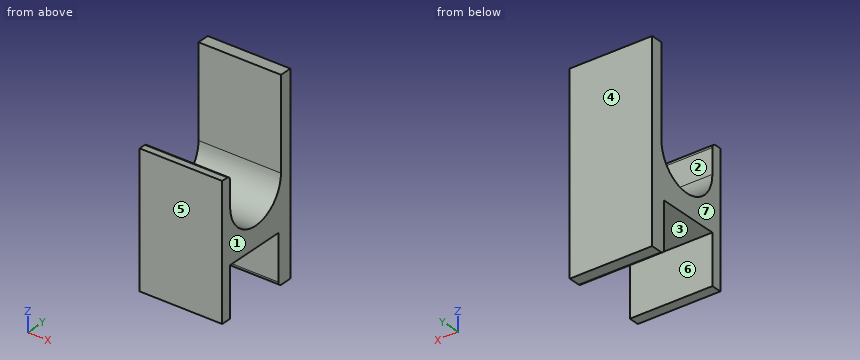
from build123d import *

# Parameters (mm, degrees)
F1_DEPTH = 25.4
F2_R     = 1.27
F3_R     = 1.27


with BuildPart() as f1:
    # F0 (on Right) → F1 (new body)
    with BuildSketch(Plane.YZ):
        with BuildLine():
            Line((-24.031516, -15.24), (-24.031516, 0))
            Line((-24.031516, 0), (-4.727516, 0))
            Line((-4.727516, 0), (-4.727516, -15.24))
            Line((-4.727516, -15.24), (0.022284, -15.24))
            Line((0.022284, -15.24), (0.022284, 44.45))
            Line((0.022284, 44.45), (-3.711516, 44.45))
            Line((-3.711516, 44.45), (-3.711516, 16.51))
            ThreePointArc((-3.711516, 16.51), (-13.871516, 6.35), (-24.031516, 16.51))
            Line((-24.031516, 16.51), (-24.031516, 25.4))
            Line((-24.031516, 25.4), (-27.206516, 25.4))
            Line((-27.206516, 25.4), (-27.206516, -15.24))
            Line((-27.206516, -15.24), (-26.082276, -15.24))
            Line((-26.082276, -15.24), (-24.031516, -15.24))
        make_face()
    extrude(amount=F1_DEPTH)

    # F2
    f2_edges = [f1.edges().sort_by_distance(p)[0] for p in [
        (12.7, -24.031516, 25.4),
    ]]
    fillet(f2_edges, radius=F2_R)

    # F3
    f3_edges = [f1.edges().sort_by_distance(p)[0] for p in [
        (12.7, -4.727516, -15.24),
    ]]
    fillet(f3_edges, radius=F3_R)


solid = f1.part
Model file for the job. Use its own axes, mm. Face numbers are marked on the shaded views. A direction names the side the tool comes from. Give positions to 0.01 mm unless a question says otherwise; leave off trailing zeros. Loops run counter-clockwise (first coordinate to the right, second up) from the corner with the lowest first, then second, coordinate; pieces in that order, holes last.
1) Saw through at D-D (z = 32.5). Write the cut outline in (x, y), plus the area to 3 significant figures.
2) Tool access for the marked faces 1, 2 and 3: list every direction of +Z, -Z, +X, -X, +Y, -Y with a clear straight run to the whole face (end or side of a thin tool).
3) Saw through at B-B (x = 16.5). Write the cut outline in (y, z).
4) Wall check: line 1 (Y direction, x = 2.75, z = -7.5); line 2 (Y direction, x = 24.5, z = 21); line 3 (Y direction, x = 8.25, z = 40.5). Give the ranges that are in metal, low to high.
5) Saw through at A-A (z = 20.5). Write the cut outline in (x, y).
6) Saw through at C-C (y = -20). Write the cut outline in (x, z).
7) Pull direction Y, two halves, no side cores. Call the marked faces 4, 5, 6 and 7: +Y half, -Y half, draft (parallel to the pull), parting line (faces both ways), or undercut.
8) Flat gauge pins, fed straight in: pin 1 Ø8 at (x, y) = (3, -21.5) entering from +Z; pin 2 Ø6 at (x, y) = (14.5, -14.5) entering from -Z. Where does each tip first touch, or does it go through?
Answer block:
1. outline: (0, -3.71) - (25.4, -3.71) - (25.4, 0.02) - (0, 0.02) - close
1. area: 94.8 mm2
2. face 1: +Z, -Z, +X, +Y, -Y
2. face 2: +Z, +X, -X
2. face 3: -Z, +X, -X
3. outline: (-27.21, -15.24) - (-24.03, -15.24) - (-24.03, 0) - (-4.73, 0) - (-4.73, -13.97) arc R1.27 ccw to (-3.46, -15.24) - (0.02, -15.24) - (0.02, 44.45) - (-3.71, 44.45) - (-3.71, 16.51) arc R10.16 cw to (-24.03, 16.51) - (-24.03, 24.13) arc R1.27 ccw to (-25.3, 25.4) - (-27.21, 25.4) - close
4. line 1: y = -27.21 to -24.03, -4.73 to 0.02
4. line 2: y = -27.21 to -24.03, -3.71 to 0.02
4. line 3: y = -3.71 to 0.02
5. outline: (0, -27.21) - (25.4, -27.21) - (25.4, -24.03) - (0, -24.03) - close; (0, -3.71) - (25.4, -3.71) - (25.4, 0.02) - (0, 0.02) - close
6. outline: (0, 0) - (25.4, 0) - (25.4, 8.41) - (0, 8.41) - close
7. face 4: +Y half
7. face 5: -Y half
7. face 6: undercut
7. face 7: draft
8. pin 1: stops at z = 25.4
8. pin 2: stops at z = 0
